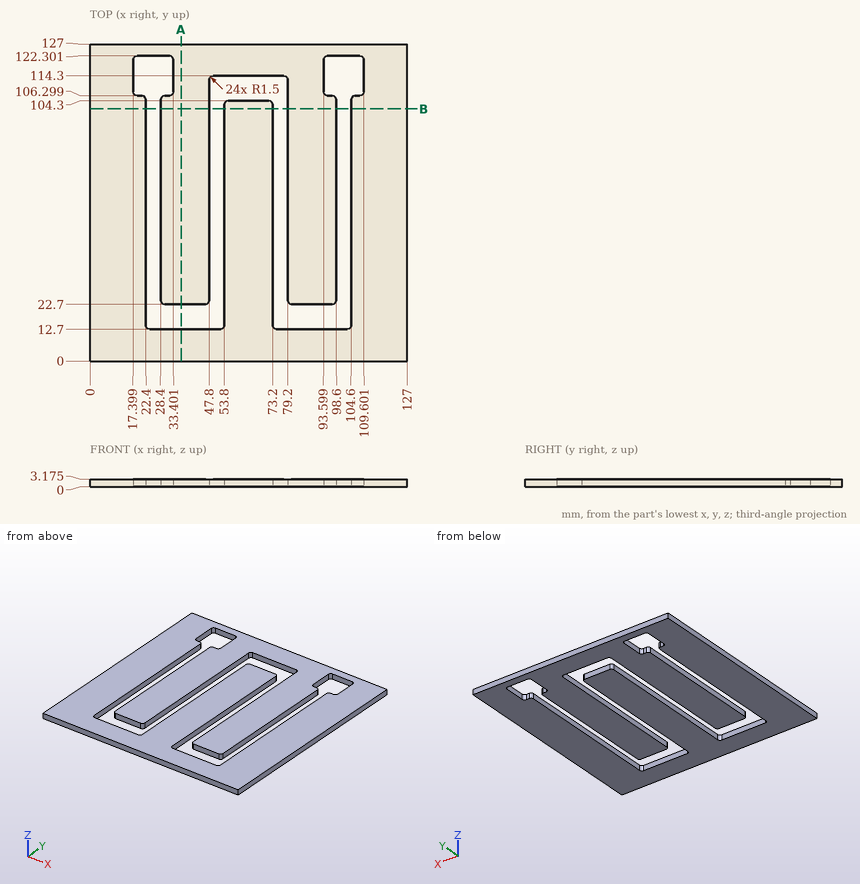
Geometry check sheet. Reference: drawing and pictorial views, mm from the part's lowest x, y, z. Coordinates: 2 decimals unless noted, no trailing zeros. Order: outer loops, then holes, each group sorted by start corner. A loop starts at its lowest first (then second) coordinate and runs counter-clockwise, first axis right, second up.
Item 1: Section check A-A (x = 36.5). Enter the section's corners in (y, z) (3 decimals).
Item 2: Scan lines: line 1 along X through (y, z) = (42, 2.35); line 2 along Y through (x, z) = (31, 1.45); line 3 along X through (y, z) = (120.5, 2.4). Record each from-to range of solid material in increasing order.
Item 3: Depth check by flat-ended pin: pin 1 (1.5 mm diameter, centred on x = 61, z = 2.5, fed in from -Y). Enter the tip coordinate at first touch or a pass-through.
Item 4: Section check B-B (y = 101). Enter the section's corners in (x, z) (3 decimals).
Check sheet entries:
1. outline: (0, 0) - (12.7, 0) - (12.7, 3.175) - (0, 3.175) - close; (22.7, 0) - (127, 0) - (127, 3.175) - (22.7, 3.175) - close
2. line 1: x = 0 to 22.4, 28.4 to 47.8, 53.8 to 73.2, 79.2 to 98.6, 104.6 to 127
2. line 2: y = 0 to 12.7, 22.7 to 106.3, 122.3 to 127
2. line 3: x = 0 to 17.4, 33.4 to 93.6, 109.6 to 127
3. pin 1: stops at y = 0
4. outline: (0, 0) - (22.4, 0) - (22.4, 3.175) - (0, 3.175) - close; (28.4, 0) - (47.8, 0) - (47.8, 3.175) - (28.4, 3.175) - close; (53.8, 0) - (73.2, 0) - (73.2, 3.175) - (53.8, 3.175) - close; (79.2, 0) - (98.6, 0) - (98.6, 3.175) - (79.2, 3.175) - close; (104.6, 0) - (127, 0) - (127, 3.175) - (104.6, 3.175) - close
